Work out the finished part from the listing and answer in its coordinate system (mm). Give positions to 0.01 mm unless a question says otherwise; leave off trailing zeros. Order: outer loops, then holes, each group sorted by start corner. A loop starts at its lowest first (then second) coordinate and runs counter-clockwise, first axis right, second up. Notation, with made-up numbers: (40, 54.5) - (49, 54.5) arc R17 ccw to (49, 82.5) - close; hole circle Ø6 at (25, 83.5). An arc over 180 degrees is marked (long way). Put each result on its own line as item: value.
```python
from build123d import *

# Parameters (mm, degrees)
SKETCH1_W                         = 4.7625
SKETCH1_H                         = 12.949588911
BOSS_EXTRUDE1_DEPTH               = 495.29818
F_1_4_0_1875_DIAMETER_HOLE1_D     = 4.7625
F_1_4_0_1875_DIAMETER_HOLE1_DEPTH = 4.7625
CHAMFER1_SIZE                     = 3.175
F_3_0MM_DOWEL_HOLE1_D             = 3.5
F_3_0MM_DOWEL_HOLE1_DEPTH         = 4.7625


with BuildPart() as part:
    # Sketch1 → Boss-Extrude1 (new body)
    with BuildSketch(Plane(origin=(0, 0, 0), x_dir=(-1, 0, 0), z_dir=(0, 0, -1))):
        with Locations((-221.207335178, 186.509282679)):
            Rectangle(SKETCH1_W, SKETCH1_H)
    extrude(amount=BOSS_EXTRUDE1_DEPTH)

    # 1/4 (0.1875) Diameter Hole1
    with Locations(Plane(origin=(223.588585178, 0, 0), x_dir=(0, 0, -1), z_dir=(1, 0, 0))):
        with Locations((12.798180471, 186.509282679)):
            Hole(F_1_4_0_1875_DIAMETER_HOLE1_D / 2, depth=F_1_4_0_1875_DIAMETER_HOLE1_DEPTH)

    # Chamfer1
    chamfer1_edges = [part.edges().sort_by_distance(p)[0] for p in [
        (218.826085178, 180.034488223, -247.64909),
        (218.826085178, 192.984077134, -247.64909),
    ]]
    chamfer(chamfer1_edges, length=CHAMFER1_SIZE)

    # Ø3.0mm Dowel Hole1
    with Locations(Plane(origin=(223.588585178, 0, 0), x_dir=(0, 0, -1), z_dir=(1, 0, 0))):
        with Locations((470.298180445, 186.509282678), (410.298180445, 186.509282678), (350.298180445, 186.509282678), (290.298180445, 186.509282678), (170.298180445, 186.509282678), (110.298180445, 186.509282678), (50.298180445, 186.509282678), (230.298180445, 186.509282678)):
            Hole(F_3_0MM_DOWEL_HOLE1_D / 2, depth=F_3_0MM_DOWEL_HOLE1_DEPTH)


solid = part.part
```
(1) Section A-A, the plane x = 220.8 is taken. Count the separate pieces of the cut face and the enclosed holes in it, then the cut area to 3 significant figures.
Geometry check:
separate pieces: 1
enclosed holes: 9
area: 5,130 mm²
(2) Straight lines are drawn through the part: line 1 (Y direction, x = 219.15, z = -471.5); line 2 (X direction, y = 192.5, z = -135); line 3 (Y direction, x = 223.1, z = -471). For each, find the intervals that lie inside material, in ascending order.
Geometry check:
line 1: y = 182.89 to 185.24, 187.78 to 190.13
line 2: x = 221.52 to 223.59
line 3: y = 180.03 to 184.91, 188.11 to 192.98
(3) Section B-B, the plane z = -164 is taken. Write down the section's boundary in (x, y).
Geometry check:
outline: (218.83, 183.21) - (222, 180.03) - (223.59, 180.03) - (223.59, 192.98) - (222, 192.98) - (218.83, 189.81) - close
(4) Given pin 1 (5.5 mm diameter, centred on y = 186.51, z = -290.3, fed in from +X); pin 2 (1.5 mm diameter, centred on x = 221, z = -195, fed in from +Y), each flat-ended and moving along its own axis, determine where each tip first touches the part or whether it passes through.
Geometry check:
pin 1: stops at x = 223.59
pin 2: stops at y = 192.73
